Here's how the part is built. I have some questions about the finished solid (model axes, mm). Face numbers are marked on the shaded views. Coordinates: 2 decimals unless noted, no trailing zeros. Write each loop counter-clockwise with the first axis right and the second up, starting at its lowest first coordinate (ties: lowest second). Pieces come first, ordered by that corner, then holes. Notation, with made-up numbers: (89, -15) - (100, -15) arc R23 cw to (100, 16) - close; hole circle Ø9 at (-2, 69.25). An arc over 180 degrees is marked (long way). Answer in a Markdown table with one row per item. Add a question column.
Item 1: I'm going to push flat-ended pins straight in: pin 1 (0.8 mm diameter, centred on y = 52, z = -28, fed in from -X); pin 2 (0.8 mm diameter, centred on y = 52, z = -1, fed in from +X); pin 3 (0.8 mm diameter, centred on x = 99.5, z = 128.5, fed in from +Y). Where does each tip first touch, or does it pass through?
Item 2: Imagine slicing it at B-B (y = 119). State how many separate pieces and enclosed holes the cut face has, plus the area to 3 significant figures.
Item 3: We'd pull the mould along Z, two halves only. Please class the marked faces 1, 2, 3 and 4: +Z half, -Z half, draft (parallel to the pull), parting line (faces both ways), or undercut.
Item 4: Imagine slicing it at A-A (x = 94.5). Please give me the cut outline in (y, z).
Item 5: If I drill on probe 1 along X at (y, z) = (60, 84.5); probe 2 along Z at (x, y) = (3.5, 69); probe 3 along X at (y, z) = (76, -50.5), over which ranges is the centre line in solid material (lowest first)? Write a range as from..to.
from build123d import *

# Parameters (mm, degrees)
EXTRUDE_THIN2_START    = -127
EXTRUDE_THIN2_DEPTH    = 254
SPLIT1_SURFACE_1_BACK  = 741.713
SPLIT1_SURFACE_1_DEPTH = 1483.426
BOSS_EXTRUDE2_DEPTH    = 2.54
BOSS_EXTRUDE3_DEPTH    = 2.54
SPLIT2_SURFACE_2_BACK  = 743.47
SPLIT2_SURFACE_2_DEPTH = 1486.94
SPLIT3_SURFACE_3_BACK  = 743.47
SPLIT3_SURFACE_3_DEPTH = 1486.94


# Read off the part's stored shape, not the designer's step: Extrude-Thin2
with BuildPart() as part:
    # Extrude-Thin2 outline → Extrude-Thin2 (new body)
    with BuildSketch(Plane.XY.offset(EXTRUDE_THIN2_START)):
        with BuildLine():
            Line((-325.542449195, 166.687822519), (-325.542449195, 166.669160537))
            Line((-325.542449195, 166.669160537), (-325.579794085, 166.687822519))
            add(Edge.make_bspline(
                [(-343.046678298, 50.863822519), (-342.854742326, 95.850869045), (-340.503085509, 136.824505781), (-325.579794085, 166.687822519)],
                knots=[0.396009693, 0.396009693, 0.396009693, 0.396009693, 0.524743478, 0.524743478, 0.524743478, 0.524743478], degree=3))
            Line((-343.046678298, 50.863822519), (343.046678298, 50.863822519))
            add(Edge.make_bspline(
                [(325.579794084, 166.687822519), (340.503085509, 136.824505781), (342.854742326, 95.850869045), (343.046678298, 50.863822519)],
                knots=[0.396009693, 0.396009693, 0.396009693, 0.396009693, 0.524743478, 0.524743478, 0.524743478, 0.524743478], degree=3))
            Line((325.579794084, 166.687822519), (323.307694442, 165.552409283))
            add(Edge.make_bspline(
                [(323.307694442, 165.552409283), (326.877593275, 158.408608594), (329.727019011, 150.576977672), (334.257221566, 133.733582984), (335.93764666, 124.722865717), (339.652297398, 96.250136339), (340.357498858, 75.350575466), (340.493401884, 53.403822519)],
                knots=[0, 0, 0, 0, 0.25, 0.25, 0.5, 0.5, 1, 1, 1, 1], degree=3))
            Line((340.493401884, 53.403822519), (-340.493401884, 53.403822519))
            add(Edge.make_bspline(
                [(-340.493401884, 53.403822519), (-340.357498858, 75.350575466), (-339.652297398, 96.250136339), (-335.937646661, 124.722865717), (-334.257221567, 133.733582984), (-329.727019012, 150.576977672), (-326.877593276, 158.408608594), (-323.307694443, 165.552409283)],
                knots=[0, 0, 0, 0, 0.5, 0.5, 0.75, 0.75, 1, 1, 1, 1], degree=3))
            Line((-323.307694443, 165.552409283), (-325.502746425, 166.649320276))
            Line((-325.502746425, 166.649320276), (-325.502746425, 166.687822519))
            Line((-325.502746425, 166.687822519), (-325.542449195, 166.687822519))
        make_face()
    extrude(amount=EXTRUDE_THIN2_DEPTH)

    # Split1: cut with a surface, the side behind it stays
    # Split1 surface: a surface, the sketch's curves swept straight by 1483.426 mm
    with BuildLine(Plane(origin=(0, 0, 0), x_dir=(0, 0, -1), z_dir=(1, 0, 0)).offset(-SPLIT1_SURFACE_1_BACK), mode=Mode.PRIVATE) as split1_surface_1_path:
        Line((-98.324088945, 166.687822519), (-97.98299712, 76.193733858))
        Line((-97.98299712, 76.193733858), (93.487324748, 76.104761498))
        Line((93.487324748, 76.104761498), (93.541066072, 166.687822519))
        Line((93.541066072, 166.687822519), (-98.324088945, 166.687822519))
    split1_surface_1 = Shell.extrude(split1_surface_1_path.wire(), (1 * SPLIT1_SURFACE_1_DEPTH, 0 * SPLIT1_SURFACE_1_DEPTH, 0 * SPLIT1_SURFACE_1_DEPTH))
    split(bisect_by=split1_surface_1, keep=Keep.BOTTOM)

    # Sketch6 → Boss-Extrude2 (add)
    with BuildSketch(Plane.XY.offset(129.54)):
        with BuildLine():
            Line((343.046678298, 50.863822519), (-343.046678298, 50.863822519))
            add(Edge.make_bspline(
                [(-325.579794085, 166.687822519), (-340.503085509, 136.824505781), (-342.854742326, 95.850869045), (-343.046678298, 50.863822519)],
                knots=[0.396009693, 0.396009693, 0.396009693, 0.396009693, 0.524743478, 0.524743478, 0.524743478, 0.524743478], degree=3))
            Line((-325.579794085, 166.687822519), (-325.542449195, 166.687822519))
            Line((-325.542449195, 166.687822519), (-299.506767133, 166.687822519))
            Line((-299.506767133, 166.687822519), (-299.506767133, 75.23611572))
            Line((-299.506767133, 75.23611572), (300.062358087, 75.23611572))
            Line((300.062358087, 75.23611572), (300.062358087, 166.687822519))
            Line((300.062358087, 166.687822519), (325.579794084, 166.687822519))
            add(Edge.make_bspline(
                [(325.579794084, 166.687822519), (340.503085509, 136.824505781), (342.854742326, 95.850869045), (343.046678298, 50.863822519)],
                knots=[0.396009693, 0.396009693, 0.396009693, 0.396009693, 0.524743478, 0.524743478, 0.524743478, 0.524743478], degree=3))
        make_face()
    extrude(amount=-BOSS_EXTRUDE2_DEPTH)

    # Sketch7 → Boss-Extrude3 (add)
    with BuildSketch(Plane(origin=(0, 0, -129.54), x_dir=(-1, 0, 0), z_dir=(0, 0, -1))):
        with BuildLine():
            Line((0, 50.863822519), (0, 75.23611572))
            Line((0, 75.23611572), (-300.062358087, 75.23611572))
            Line((-300.062358087, 75.23611572), (-300.062358087, 166.687822519))
            Line((-300.062358087, 166.687822519), (-325.502746425, 166.687822519))
            Line((-325.502746425, 166.687822519), (-325.542449195, 166.687822519))
            Line((-325.542449195, 166.687822519), (-325.579794085, 166.687822519))
            add(Edge.make_bspline(
                [(-325.579794085, 166.687822519), (-340.503085509, 136.824505781), (-342.854742326, 95.850869045), (-343.046678298, 50.863822519)],
                knots=[0.396009693, 0.396009693, 0.396009693, 0.396009693, 0.524743478, 0.524743478, 0.524743478, 0.524743478], degree=3))
            Line((-343.046678298, 50.863822519), (0, 50.863822519))
        make_face()
        with BuildLine():
            Line((299.506767133, 75.23611572), (0, 75.23611572))
            Line((0, 75.23611572), (0, 50.863822519))
            Line((0, 50.863822519), (343.046678298, 50.863822519))
            add(Edge.make_bspline(
                [(325.579794084, 166.687822519), (340.503085509, 136.824505781), (342.854742326, 95.850869045), (343.046678298, 50.863822519)],
                knots=[0.396009693, 0.396009693, 0.396009693, 0.396009693, 0.524743478, 0.524743478, 0.524743478, 0.524743478], degree=3))
            Line((325.579794084, 166.687822519), (299.506767133, 166.687822519))
            Line((299.506767133, 166.687822519), (299.506767133, 75.23611572))
        make_face()
    extrude(amount=-BOSS_EXTRUDE3_DEPTH)

    # Split2: cut with a surface, the side it looks to stays
    # Split2 surface: a surface, the sketch's curves swept straight by 1486.94 mm
    with BuildLine(Plane(origin=(0, 0, 0), x_dir=(1, 0, 0), z_dir=(0, 1, 0)).offset(-SPLIT2_SURFACE_2_BACK), mode=Mode.PRIVATE) as split2_surface_2_path:
        Line((-317.646678298, 104.14), (317.080123639, 104.14))
        Line((317.080123639, 104.14), (317.080123639, -104.14))
        Line((317.080123639, -104.14), (-317.646678298, -104.14))
        Line((-317.646678298, -104.14), (-317.646678298, 104.14))
    split2_surface_2 = Shell.extrude(split2_surface_2_path.wire(), (0 * SPLIT2_SURFACE_2_DEPTH, 1 * SPLIT2_SURFACE_2_DEPTH, 0 * SPLIT2_SURFACE_2_DEPTH))
    split(bisect_by=split2_surface_2, keep=Keep.TOP)

    # Split3: cut with a surface, the side behind it stays
    # Split3 surface: a surface, the sketch's curves swept straight by 1486.94 mm
    with BuildLine(Plane(origin=(0, 0, 0), x_dir=(0, 0, -1), z_dir=(1, 0, 0)).offset(-SPLIT3_SURFACE_3_BACK), mode=Mode.PRIVATE) as split3_surface_3_path:
        Line((-165.841686169, 137.985822519), (168.310027545, 137.985822519))
    split3_surface_3 = Shell.extrude(split3_surface_3_path.wire(), (1 * SPLIT3_SURFACE_3_DEPTH, 0 * SPLIT3_SURFACE_3_DEPTH, 0 * SPLIT3_SURFACE_3_DEPTH))
    split(bisect_by=split3_surface_3, keep=Keep.BOTTOM)


solid = part.part
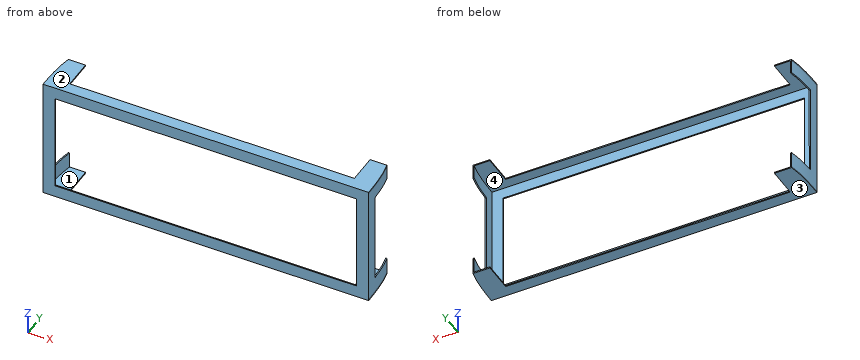
Here are the results:
| question | item | result |
|---|---|---|
| 1 | pin 1 | stops at x = -343.04 |
| 1 | pin 2 | stops at x = 343.04 |
| 1 | pin 3 | stops at y = 75.24 |
| 2 | separate pieces | 4 |
| 2 | enclosed holes | 0 |
| 2 | area | 721 mm2 |
| 3 | face 1 | undercut |
| 3 | face 2 | +Z half |
| 3 | face 3 | -Z half |
| 3 | face 4 | undercut |
| 4 | outline | (50.86, -129.54) - (75.24, -129.54) - (75.24, -127) - (53.4, -127) - (53.4, -104.14) - (50.86, -104.14) - close; (50.86, 104.14) - (53.4, 104.14) - (53.4, 127) - (75.24, 127) - (75.24, 129.54) - (50.86, 129.54) - close |
| 5 | probe 1 | x = -342.97..-340.43, 340.43..342.97 |
| 5 | probe 2 | z = -129.54..-127, 127..129.54 |
| 5 | probe 3 | x = -342.63..-340.09, 340.09..342.63 |
